Check sheet for the modelled part. Datum: model origin and axes. Units: mm. Face numbers are marked on the shaded views. Give positions to 0.01 mm unless a question says otherwise; leave off trailing zeros. Order: outer loops, then holes, each group sorted by start corner. A loop starts at its lowest first (then second) coordinate and runs counter-clockwise, first axis right, second up. Notation, with made-up numbers: M 64,48 L 74,48 A27 ccw 74,82 Z; hole C 71.5,-13.75 d3. An arc over 180 degrees is marked long. Return JSON: item names as keys, results as strings. Group by question number.
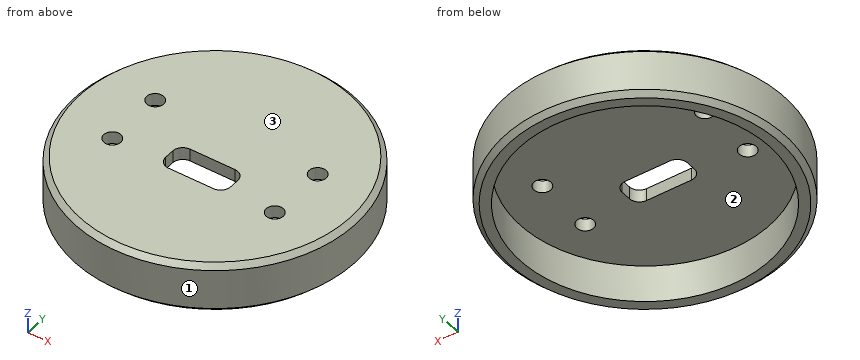
from build123d import *

# Parameters (mm, degrees)
SKETCH_1_R          = 28
EXTRUDE_1_DEPTH     = 10
SKETCH_3_R          = 25
CUT_EXTRUDE_2_DEPTH = 7.5
CUT_EXTRUDE_4_REACH = 42.302
SKETCH_6_W          = 13
SKETCH_6_H          = 6
FILLET_3_R          = 2
HOLE_WIZARD_M31_D   = 3.4
CHAMFER_1_SIZE      = 1


with BuildPart() as part:
    # Эскиз1 → Бобышка-Вытянуть1 (new body)
    with BuildSketch(Plane.XY):
        Circle(SKETCH_1_R)
    extrude(amount=EXTRUDE_1_DEPTH)

    # Эскиз3 → Вырез-Вытянуть2 (cut)
    with BuildSketch(Plane(origin=(0, 0, 0), x_dir=(-1, 0, 0), z_dir=(0, 0, -1))):
        Circle(SKETCH_3_R)
    extrude(amount=-CUT_EXTRUDE_2_DEPTH, mode=Mode.SUBTRACT)

    # Эскиз6 → Вырез-Вытянуть4 (cut, up to next)
    with BuildSketch(Plane(origin=(0, 0, 7.5), x_dir=(-1, 0, 0), z_dir=(0, 0, -1)), mode=Mode.PRIVATE) as cut_extrude_4_sk1:
        with Locations((-0.103380177, -3.86)):
            Rectangle(SKETCH_6_W, SKETCH_6_H)
    cut_extrude_4_tool1 = extrude(cut_extrude_4_sk1.sketch, amount=-CUT_EXTRUDE_4_REACH, mode=Mode.PRIVATE) & part.part
    add(cut_extrude_4_tool1.solids().sort_by_distance((0.10338, -3.86, 7.5))[0], mode=Mode.SUBTRACT)

    # Скругление3
    fillet_3_edges = [part.edges().sort_by_distance(p)[0] for p in [
        (-6.396619823, -0.86, 8.75),
        (-6.396619823, -6.86, 8.75),
        (6.603380177, -6.86, 8.75),
        (6.603380177, -0.86, 8.75),
    ]]
    fillet(fillet_3_edges, radius=FILLET_3_R)

    # Отверстие с зазором M31 (through all)
    with Locations(Plane(origin=(0, 0, 7.5), x_dir=(-1, 0, 0), z_dir=(0, 0, -1))):
        with Locations((16.25, -6), (16.25, 6), (-16.25, 6), (-16.25, -6)):
            Hole(HOLE_WIZARD_M31_D / 2)

    # Фаска1
    chamfer_1_edges = [part.edges().sort_by_distance(p)[0] for p in [
        (-28, 0, 0),
        (-28, 0, 10),
    ]]
    chamfer(chamfer_1_edges, length=CHAMFER_1_SIZE)


solid = part.part
1) Depth check by flat-ended pin: P1, Ø4, axis at x = -16.25, y = -6, coming from the -Z side; P2, Ø2, axis at x = 2, z = 8.5, coming from the +Y side; P3, Ø5, axis at x = -10, z = 7.5, coming from the -Y side; P4, Ø2.5, axis at x = 16.25, y = -6, coming from the +Z side. Enter the tip coordinate at first touch or a pass-through.
2) Sectioned sample at A-A on x = 0. Record the boundary of the cut face in (y, z), then the cut area to 3 significant figures.
3) Sectioned sample at B-B on y = 0. Record the boundary of the cut face in (x, z), then the cut area to 3 significant figures.
4) Release check for a two-part mould opening along Y. For the marked faces 1, 2 and 3 record: released by +Y, released by -Y, zero draft, split by the parting line, or undercut.
5) Sectioned sample at C-C on y = -6. State how many separate pieces and enclosed holes the cut face has, then the cut area to 3 significant figures.
6) Material ranges on line 1 along Y through (x, z) = (0, 2); line 2 along Y through (x, z) = (-16.25, 9.2); line 3 along Y through (x, z) = (-16.25, 9.45), recorded low to high.
Reply:
{
 "1": {"P1": "z = 7.5", "P2": "y = 27.98", "P3": "y = -26.98", "P4": "through"},
 "2": {"outline": "M -28,1 L -27,0 L -25,0 L -25,7.5 L -6.86,7.5 L -6.86,10 L -27,10 L -28,9 Z; M -0.86,7.5 L 25,7.5 L 25,0 L 27,0 L 28,1 L 28,9 L 27,10 L -0.86,10 Z", "area": "168 mm^2"},
 "3": {"outline": "M -28,1 L -27,0 L -25,0 L -25,7.5 L 25,7.5 L 25,0 L 27,0 L 28,1 L 28,9 L 27,10 L -27,10 L -28,9 Z", "area": "183 mm^2"},
 "4": {"face 1": "split by the parting line", "face 2": "undercut", "face 3": "zero draft"},
 "5": {"separate pieces": "4", "enclosed holes": "0", "area": "133 mm^2"},
 "6": {"line 1": "-28 to -25, 25 to 28", "line 2": "-22.56 to -7.7, -4.3 to 4.3, 7.7 to 22.56", "line 3": "-22.25 to -7.7, -4.3 to 4.3, 7.7 to 22.25"}
}
